```python
from build123d import *

# Parameters (mm, degrees)
SKETCH1_R      = 2
SKETCH1_R_2    = 3.3
SKETCH1_R_3    = 3.2
EXTRUDE1_DEPTH = 3.175


with BuildPart() as part:
    # Sketch1 → Extrude1 (new body)
    with BuildSketch(Plane.XY):
        with BuildLine():
            Line((138.1125, 191.25), (138.1125, -191.25))
            ThreePointArc((138.1125, -191.25), (0, -196.183512306), (-138.1125, -191.25))
            Line((-138.1125, -191.25), (-138.1125, 191.25))
            ThreePointArc((-138.1125, 191.25), (0, 196.183512306), (138.1125, 191.25))
        make_face()
        with Locations((46.1772, 82.55)):
            Circle(SKETCH1_R, mode=Mode.SUBTRACT)
        with Locations((53, 184.28)):
            Circle(SKETCH1_R_2, mode=Mode.SUBTRACT)
        with Locations((-24.13, 139.446)):
            Circle(SKETCH1_R, mode=Mode.SUBTRACT)
        with Locations((-133.096, 104.936568767)):
            Circle(SKETCH1_R, mode=Mode.SUBTRACT)
        with Locations((-53, 184.28)):
            Circle(SKETCH1_R_2, mode=Mode.SUBTRACT)
        with Locations((0, 43)):
            Circle(SKETCH1_R_3, mode=Mode.SUBTRACT)
        with Locations((0, 5.15)):
            Circle(SKETCH1_R_2, mode=Mode.SUBTRACT)
        with Locations((0, -36.65)):
            Circle(SKETCH1_R_2, mode=Mode.SUBTRACT)
        with Locations((133.096, 12.7)):
            Circle(SKETCH1_R, mode=Mode.SUBTRACT)
        with Locations((133.096, -76.2)):
            Circle(SKETCH1_R, mode=Mode.SUBTRACT)
        with Locations((98.425, -139.446)):
            Circle(SKETCH1_R, mode=Mode.SUBTRACT)
        with Locations((70, -175.85)):
            Circle(SKETCH1_R_2, mode=Mode.SUBTRACT)
        with Locations((-3.175, -139.446)):
            Circle(SKETCH1_R, mode=Mode.SUBTRACT)
        with Locations((-133.096, -98.263431233)):
            Circle(SKETCH1_R, mode=Mode.SUBTRACT)
        with Locations((-104.775, -139.446)):
            Circle(SKETCH1_R, mode=Mode.SUBTRACT)
        with Locations((-70, -175.85)):
            Circle(SKETCH1_R_3, mode=Mode.SUBTRACT)
    extrude(amount=EXTRUDE1_DEPTH)


solid = part.part
```
The model under review builds one solid part; all positions refer to its coordinate system, in mm. Round coordinates to 2 decimals unless told otherwise and drop trailing zeros. Order: outer loops, then holes, each group sorted by start corner. A loop starts at its lowest first (then second) coordinate and runs counter-clockwise, first axis right, second up.
Item 1: Add section A-A, the plane x = -111. State the section outline as (y, z) points (3 decimals), and give its area (3 significant figures).
Working result:
outline: (-192.998, 0) - (192.998, 0) - (192.998, 3.175) - (-192.998, 3.175) - close
area: 1,230 mm2
Item 2: To check wall thickness, follow probe 1 along X at (y, z) = (184.28, 2.35); probe 2 along Y at (x, z) = (-23, 1.45); probe 3 along Y at (x, z) = (-52, 1.85). State the ranges of each line that lie inside material, in increasing order.
Working result:
probe 1: x = -138.11 to -56.3, -49.7 to 49.7, 56.3 to 138.11
probe 2: y = -196.05 to 137.8, 141.1 to 196.05
probe 3: y = -195.48 to 181.14, 187.42 to 195.48
Item 3: For pin 1 (2.5 mm diameter, centred on x = 133.096, y = -76.2, fed in from +Z), flat-tipped, find the tip position at first contact; note if it passes through.
Working result:
pin 1: passes through
